Autodesk Inventor part; units mm, degrees
ref_plane "YZ Plane" through (0, 0, 0) normal (1, 0, 0) x (0, 1, 0)
ref_plane "XY Plane" through (0, 0, 0) normal (0, 0, 1) x (1, 0, 0)
sketch "Sketch1" plane through (0, 0, 0) normal (0, 1, 0) x (-1, 0, 0)
  line L0 (-149.225, 149.225) -> (149.225, 149.225)
  line L1 (149.225, 149.225) -> (149.225, -149.225)
  line L2 (149.225, -149.225) -> (-149.225, -149.225)
  line L3 (-149.225, -149.225) -> (-149.225, 149.225)
  line L4 (-149.225, 149.225) -> (149.225, -149.225) construction
  line L5 (149.225, 149.225) -> (-149.225, -149.225) construction
  point P0 (0, 0)
  dimension "d0" = 298.45
  dimension "d1" = 298.45
ref_plane "Work Plane1" through (0, 165.1, 0) normal (0, 1, 0) x (-1, 0, 0)
sketch "Sketch2" plane through (0, 165.1, 0) normal (0, 1, 0) x (-1, 0, 0)
  line L0 (-31.75, 31.75) -> (31.75, 31.75)
  line L1 (31.75, 31.75) -> (31.75, -31.75)
  line L2 (31.75, -31.75) -> (-31.75, -31.75)
  line L3 (-31.75, -31.75) -> (-31.75, 31.75)
  line L4 (-31.75, 31.75) -> (31.75, -31.75) construction
  line L5 (31.75, 31.75) -> (-31.75, -31.75) construction
  point P0 (0, 0)
  dimension "d3" = 63.5
  dimension "d4" = 63.5
loft "Loft1" add profiles "Sketch2", "Sketch1"
shell "Shell1" thickness 2.54 removed faces 1 at (-49.7417, 0, -49.7417)
properties part number "hologram pyramid (for assembly)"
Read the model definition and answer for the solid it produces. Units are mm, in the model's axes. Give positions to 0.01 mm unless a question says otherwise; leave off trailing zeros.
Item 1: Each of these flat-tipped pins is pushed along its axis until it touches: pin 1 Ø12 at (x, z) = (86, 13) entering from +Y; pin 2 Ø3 at (x, y) = (48.5, 28) entering from -Z; pin 3 Ø5 at (y, z) = (94, -71) entering from -X. Where does it stop, or does it pass through?
Item 2: Find the intervals of material crossed by line 1 along X through (y, z) = (68.5, 64.5); line 2 along Z through (x, y) = (79.5, 40); line 3 along X through (y, z) = (71, -14.5), in increasing order.
Item 3: The mould has two halves that part along X. Classify faces 1 (the flat face through (0, 165.1, 1)), 2 (the flat face through (0, 162.56, 1)): released by +X, released by -X, zero draft, split by the parting line, or undercut.
Taken from the geometry:
1. pin 1: stops at y = 97.29
1. pin 2: stops at z = -130.37
1. pin 3: stops at x = -84.12
2. line 1: x = -100.48 to -97.37, 97.37 to 100.48
2. line 2: z = -120.76 to -117.65, 117.65 to 120.76
2. line 3: x = -98.71 to -95.59, 95.59 to 98.71
3. face 1: zero draft
3. face 2: undercut
